from build123d import *

# Parameters (mm, degrees)
SKETCH_1_W          = 15
SKETCH_1_H          = 15
SKETCH_1_R          = 5.5
EXTRUDE_1_DEPTH     = 45
SKETCH_5_W          = 15
SKETCH_5_H          = 15
EXTRUDE_3_DEPTH     = 15
FILLET_2_R          = 7.5
SKETCH_6_R          = 2.1
CUT_EXTRUDE_1_DEPTH = 49.023431781
CUT_EXTRUDE_2_DEPTH = 8
SKETCH_9_W          = 8
SKETCH_9_H          = 8
SKETCH_9_R          = 1.6
EXTRUDE_4_DEPTH     = 7
FILLET_3_R          = 2
SKETCH_11_R         = 3.2
CUT_EXTRUDE_3_DEPTH = 3.75


with BuildPart() as part:
    # ｽｹｯﾁ1 → ﾎﾞｽ - 押し出し1 (new body)
    with BuildSketch(Plane.XY):
        Rectangle(SKETCH_1_W, SKETCH_1_H)
        with Locations(Location((0, 0, 0), (0, 0, 180))):
            Circle(SKETCH_1_R, mode=Mode.SUBTRACT)
    extrude(amount=EXTRUDE_1_DEPTH)

    # ｽｹｯﾁ5 → ﾎﾞｽ - 押し出し3 (add)
    with BuildSketch(Plane.XY.offset(45)):
        Rectangle(SKETCH_5_W, SKETCH_5_H)
    extrude(amount=-EXTRUDE_3_DEPTH)

    # ﾌｨﾚｯﾄ2
    fillet_2_edges = [part.edges().sort_by_distance(p)[0] for p in [
        (0, -7.5, 45),
        (0, 7.5, 45),
    ]]
    fillet(fillet_2_edges, radius=FILLET_2_R - 0.0001)  # a hair under: the kernel refuses the full size

    # ｽｹｯﾁ6 → ｶｯﾄ - 押し出し1 (cut, through all)
    with BuildSketch(Plane(origin=(7.5, 0, 0), x_dir=(0, 0, -1), z_dir=(1, 0, 0))):
        with Locations((-37.5, 0)):
            Circle(SKETCH_6_R)
    extrude(amount=-CUT_EXTRUDE_1_DEPTH, mode=Mode.SUBTRACT)

    # ｽｹｯﾁ7 → ｶｯﾄ - 押し出し2 (cut)
    with BuildSketch(Plane(origin=(7.5, 0, 0), x_dir=(0, 0, -1), z_dir=(1, 0, 0))):
        with BuildLine():
            Line((-37.5, -9.5), (2, -9.5))
            Line((2, -9.5), (2, 9.5))
            Line((2, 9.5), (-37.5, 9.5))
            ThreePointArc((-37.5, 9.5), (-44.217514421, 6.717514421), (-47, 0))
            ThreePointArc((-47, 0), (-44.217514421, -6.717514421), (-37.5, -9.5))
        make_face()
    extrude(amount=-CUT_EXTRUDE_2_DEPTH, mode=Mode.SUBTRACT)

    # ｽｹｯﾁ9 → ﾎﾞｽ - 押し出し4 (add)
    # profile 1 of 4: a face of its own
    with BuildSketch(Plane(origin=(-0.5, 0, 0), x_dir=(0, 0, -1), z_dir=(1, 0, 0))):
        with Locations((-4, -9.477225575)):
            Rectangle(SKETCH_9_W, SKETCH_9_H)
        with Locations((-4, -9.477225575)):
            Circle(SKETCH_9_R, mode=Mode.SUBTRACT)
    # profile 2 of 4: a face of its own
    with BuildSketch(Plane(origin=(-0.5, 0, 0), x_dir=(0, 0, -1), z_dir=(1, 0, 0))):
        with Locations((-26, 9.477225575)):
            Rectangle(SKETCH_9_W, SKETCH_9_H)
        with Locations((-26, 9.477225575)):
            Circle(SKETCH_9_R, mode=Mode.SUBTRACT)
    # profile 3 of 4: a face of its own
    with BuildSketch(Plane(origin=(-0.5, 0, 0), x_dir=(0, 0, -1), z_dir=(1, 0, 0))):
        with Locations((-4, 9.477225575)):
            Rectangle(SKETCH_9_W, SKETCH_9_H)
        with Locations((-4, 9.477225575)):
            Circle(SKETCH_9_R, mode=Mode.SUBTRACT)
    # profile 4 of 4: a face of its own
    with BuildSketch(Plane(origin=(-0.5, 0, 0), x_dir=(0, 0, -1), z_dir=(1, 0, 0))):
        with Locations((-26, -9.477225575)):
            Rectangle(SKETCH_9_W, SKETCH_9_H)
        with Locations((-26, -9.477225575)):
            Circle(SKETCH_9_R, mode=Mode.SUBTRACT)
    extrude(amount=-EXTRUDE_4_DEPTH)

    # ﾌｨﾚｯﾄ3
    fillet_3_edges = [part.edges().sort_by_distance(p)[0] for p in [
        (-4, 13.477225575, 22),
        (-4, 7.5, 30),
        (-4, 13.477225575, 30),
        (-4, 7.5, 22),
        (-4, 13.477225575, 0),
        (-4, 7.5, 8),
        (-4, 13.477225575, 8),
        (-4, -13.477225575, 30),
        (-4, -7.5, 22),
        (-4, -13.477225575, 22),
        (-4, -7.5, 30),
        (-4, -13.477225575, 8),
        (-4, -13.477225575, 0),
        (-4, -7.5, 8),
    ]]
    fillet(fillet_3_edges, radius=FILLET_3_R)

    # ｽｹｯﾁ11 → ｶｯﾄ - 押し出し3 (cut)
    with BuildSketch(Plane.ZY.offset(7.5)):
        with Locations((4, 9.477225575)):
            Circle(SKETCH_11_R)
        with Locations((26, 9.477225575)):
            Circle(SKETCH_11_R)
        with Locations((26, -9.477225575)):
            Circle(SKETCH_11_R)
        with Locations((4, -9.477225575)):
            Circle(SKETCH_11_R)
    extrude(amount=-CUT_EXTRUDE_3_DEPTH, mode=Mode.SUBTRACT)


solid = part.part
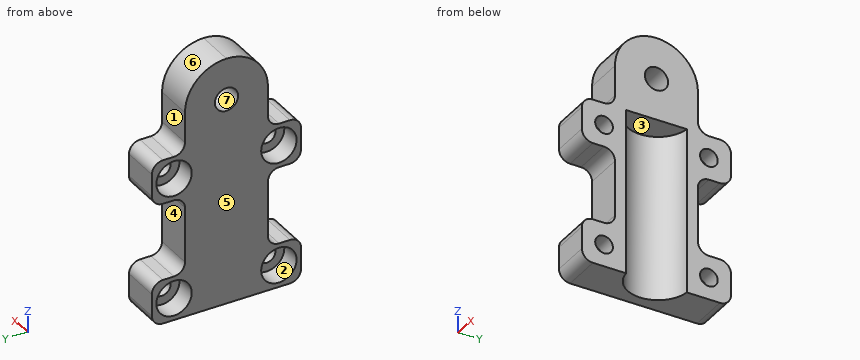
Geometry check sheet. Reference: the model listing, model coordinates, mm. Face numbers are marked on the shaded views. A direction names the side the tool comes from. Round coordinates to 2 decimals unless told otherwise and drop trailing zeros. Order: outer loops, then holes, each group sorted by start corner. A loop starts at its lowest first (then second) coordinate and runs counter-clockwise, first axis right, second up. Notation, with made-up numbers: (48.5, 54) - (74.5, 54) arc R26 ccw to (74.5, 82) - close; hole circle Ø8 at (10, -17). An arc over 180 degrees is marked (long way). One line per question, with ' | ' between items. Start each with the question number.
(1) Depth check by flat-ended pin: pin 1 Ø3.5 at (y, z) = (-9.48, 26) entering from -X; pin 2 Ø3 at (x, y) = (-5, 9.5) entering from +Z; pin 3 Ø0.6 at (x, y) = (-3.5, -10.5) entering from +Z; pin 4 Ø3 at (y, z) = (9.48, 4) entering from -X. Enter the tip coordinate at first touch or a pass-through.
(2) Sectioned sample at D-D on z = 27. Record the cut outline in (x, y), and give its area (3 significant figures).
(3) Sectioned sample at C-C on y = 4. Record the cut outline in (x, z), and give its area (3 significant figures).
(4) Sectioned sample at A-A on z = 4. Record the cut outline in (x, y), and give its area (3 significant figures).
(5) Release check for a two-part mould opening along Z. For the marked faces 5, 6 and 7 record: released by +Z, released by -Z, zero draft, split by the parting line, or undercut.
(6) Thickness scan on L1, parallel to Y at x = -5.85, z = 26; L2, parallel to Z at x = -1.25, y = 9.5; L3, parallel to Y at x = -4, z = 28.5. Record the ranges inside material, lowest first. Write a range as [from, to].
(7) Sectioned sample at B-B on z = 14.5. Record the cut outline in (x, y), and give its area (3 significant figures).
(8) Access from +Z, -Z, +X, -X, +Y, -Y to the whole of each face (thin tool, end or side, straight path). Record for the marked faces 1, 2, 3 and 4.
Conclusion:
1) pin 1: stops at x = -3.75 | pin 2: stops at z = 30.68 | pin 3: stops at z = 30 | pin 4: passes through
2) outline: (-7.5, -13.48) - (-0.5, -13.48) - (-0.5, -10.73) - (-3.75, -10.73) - (-3.75, -12.52) - (-7.5, -12.52) - close; (-7.5, -6.44) - (-3.75, -6.44) - (-3.75, -8.23) - (-0.5, -8.23) - (-0.5, -5.48) arc R5.5 cw to (-0.5, 5.48) - (-0.5, 8.23) - (-3.75, 8.23) - (-3.75, 6.44) - (-7.5, 6.44) - close; (-7.5, 12.52) - (-3.75, 12.52) - (-3.75, 10.73) - (-0.5, 10.73) - (-0.5, 13.48) - (-7.5, 13.48) - close | area: 84.8 mm2
3) outline: (-7.5, 0) - (-3.77, 0) - (-3.77, 30) - (-0.5, 30) - (-0.5, 43.84) - (-7.5, 43.84) - close | area: 209 mm2
4) outline: (-7.5, -13.48) - (-0.5, -13.48) - (-0.5, -11.08) - (-3.75, -11.08) - (-3.75, -12.68) - (-7.5, -12.68) - close; (-7.5, -6.28) - (-3.75, -6.28) - (-3.75, -7.88) - (-0.5, -7.88) - (-0.5, -5.48) arc R5.5 cw to (-0.5, 5.48) - (-0.5, 7.88) - (-3.75, 7.88) - (-3.75, 6.28) - (-7.5, 6.28) - close; (-7.5, 12.68) - (-3.75, 12.68) - (-3.75, 11.08) - (-0.5, 11.08) - (-0.5, 13.48) - (-7.5, 13.48) - close | area: 77.9 mm2
5) face 5: zero draft | face 6: released by +Z | face 7: undercut
6) L1: y = [-13.48, -12.68], [-6.28, 6.28], [12.68, 13.48] | L2: z = [0, 2.4], [5.6, 8], [22, 24.4], [27.6, 30] | L3: y = [-13.41, -11.47], [-7.48, -3.77], [3.77, 7.48], [11.47, 13.41]
7) outline: (-7.5, -7.5) - (-0.5, -7.5) - (-0.5, -5.48) arc R5.5 cw to (-0.5, 5.48) - (-0.5, 7.5) - (-7.5, 7.5) - close | area: 63.0 mm2
8) face 1: +Z, +X, -X, +Y | face 2: -X | face 3: -Z, +X | face 4: +X, -X, +Y
